Work out the finished part from the listing and answer in its coordinate system (mm). Coordinates: 2 decimals unless noted, no trailing zeros. Loops run counter-clockwise (first coordinate to the right, second up) from the corner with the lowest first, then second, coordinate; pieces in that order, holes last. Notation, with made-up numbers: (42.5, -29) - (75.5, -29) arc R16 cw to (75.5, 0) - close; hole circle Ø10 at (27, 19.25). An arc over 180 degrees is marked (long way). Write each question's results on one line, items separated by ' | '. Start each with the question number.
Item 1: Consider probe 1 along X at (y, z) = (-1.5, 46.5); probe 2 along Y at (x, z) = (100, 54); probe 3 along Z at (x, y) = (105, -7.5). Determine where each line is inside the solid, lowest interval first. Write a range as [from, to].
Item 2: Each of these flat-tipped pins is pushed along its axis until it touches: pin 1 Ø3 at (x, z) = (83, 39.5) entering from -Y; pin 2 Ø1 at (x, z) = (96, 56.5) entering from +Y; pin 3 Ø2 at (y, z) = (-2.5, 64) entering from +X; pin 4 Ø10 at (y, z) = (-1, 54) entering from +X. Where does it stop, or does it pass through?
Item 3: Section A-A, the plane z = 14 is taken. Write down the section's boundary in (x, y).
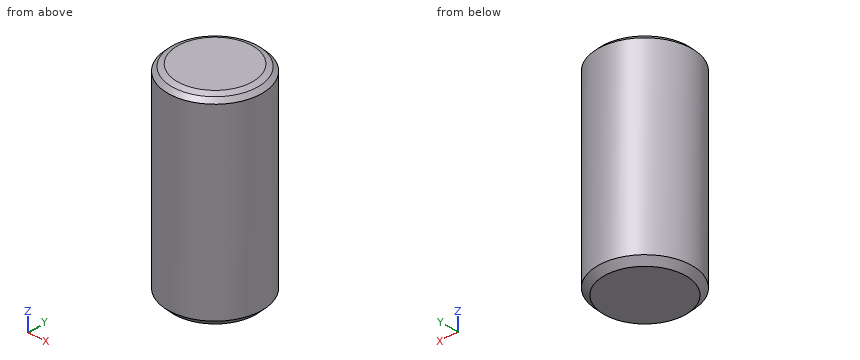
from build123d import *

# Parameters (mm, degrees)
F0_R     = 15
F1_DEPTH = 32
F2_SIZE  = 2
F3_SIZE  = 1


with BuildPart() as f1:
    # F0 (on Top) → F1 (new body, symmetric)
    with BuildSketch(Plane.XY):
        with Locations((95, 0)):
            Circle(F0_R)
    extrude(amount=F1_DEPTH, both=True)

    # F2
    f2_edges = [f1.edges().sort_by_distance(p)[0] for p in [
        (80, 0, 32),
        (80, 0, -32),
    ]]
    chamfer(f2_edges, length=F2_SIZE)

    # F3
    f3_edges = [f1.edges().sort_by_distance(p)[0] for p in [
        (82, 0, 32),
    ]]
    chamfer(f3_edges, length=F3_SIZE)


with BuildPart() as f1_1:
    # F4: moved
    add(f1.part.moved(Location((0, 0, 40))))


solid = f1_1.part
Answer key:
1) probe 1: x = [80.08, 109.92] | probe 2: y = [-14.14, 14.14] | probe 3: z = [8, 71.79]
2) pin 1: stops at y = -10.71 | pin 2: stops at y = 14.99 | pin 3: stops at x = 109.92 | pin 4: stops at x = 110
3) outline: circle Ø30 at (95, 0)
